Can you work these out from the model? Positions are in its coordinate system, mm. A direction names the side the tool comes from. Give positions to 0.01 mm unless a question says otherwise; leave off trailing zeros. Loops run counter-clockwise (first coordinate to the right, second up) from the corner with the lowest first, then second, coordinate; pieces in that order, holes last. Notation, with made-up numbers: M 49,33 L 91,33 A24 cw 91,52 Z; hole C 25.5,86 d8. An arc over 180 degrees is marked long. Answer as a JSON object with one key per item and string values.
```python
from build123d import *

# Parameters (mm, degrees)
SKETCH1_W           = 16.65
SKETCH1_H           = 12
BOSS_EXTRUDE1_DEPTH = 13
SKETCH2_W           = 7
SKETCH2_H           = 10.524951481
CUT_EXTRUDE1_DEPTH  = 13
SKETCH3_W           = 6.35563947
SKETCH3_H           = 6.957033312
SKETCH3_W_2         = 6.600584973
SKETCH3_H_2         = 6.806684851
BOSS_EXTRUDE2_DEPTH = 1
SKETCH4_R           = 2.546367572
SKETCH4_R_2         = 2.582102571
BOSS_EXTRUDE3_DEPTH = 1.5
FILLET1_R           = 1


with BuildPart() as part:
    # Sketch1 → Boss-Extrude1 (new body)
    with BuildSketch(Plane(origin=(0, 0, 0), x_dir=(1, 0, 0), z_dir=(0, 1, 0))):
        with Locations((-0.458958652, 0.629402757)):
            Rectangle(SKETCH1_W, SKETCH1_H)
    extrude(amount=BOSS_EXTRUDE1_DEPTH)

    # Sketch2 → Cut-Extrude1 (cut)
    with BuildSketch(Plane.XY.offset(5.370597243)):
        with Locations((-4.283958652, 12.062475741)):
            Rectangle(SKETCH2_W, SKETCH2_H)
        with Locations((3.366041348, 12.062475741)):
            Rectangle(SKETCH2_W, SKETCH2_H)
    extrude(amount=-CUT_EXTRUDE1_DEPTH, mode=Mode.SUBTRACT)

    # Sketch3 → Boss-Extrude2 (add)
    with BuildSketch(Plane(origin=(0, 6.8, 0), x_dir=(1, 0, 0), z_dir=(0, 1, 0))):
        with Locations((-4.190334083, 0.759249154)):
            Rectangle(SKETCH3_W, SKETCH3_H)
        with Locations((3.300292487, 0.834423384)):
            Rectangle(SKETCH3_W_2, SKETCH3_H_2)
    extrude(amount=BOSS_EXTRUDE2_DEPTH)

    # Sketch4 → Boss-Extrude3 (add)
    with BuildSketch(Plane(origin=(0, 7.8, 0), x_dir=(1, 0, 0), z_dir=(0, 1, 0))):
        with Locations((-4.183500062, 0.684074924)):
            Circle(SKETCH4_R)
        with Locations((3.456935343, 0.793419259)):
            Circle(SKETCH4_R_2)
    extrude(amount=BOSS_EXTRUDE3_DEPTH)

    # Fillet1
    fillet1_edges = [part.edges().sort_by_distance(p)[0] for p in [
        (-6.729867634, 9.3, -0.684074924),
        (0.874832772, 9.3, -0.793419259),
    ]]
    fillet(fillet1_edges, radius=FILLET1_R)


solid = part.part
```
1) Suppose I cut it at A-A, the plane y = 10.5. Write out the boundary of the cut face in (x, z), and give its area (3 significant figures).
Answer list:
{"outline": "M -8.78,-6.63 L -7.78,-6.63 L -7.78,5.37 L -8.78,5.37 Z; M -0.78,-6.63 L -0.13,-6.63 L -0.13,5.37 L -0.78,5.37 Z; M 6.87,-6.63 L 7.87,-6.63 L 7.87,5.37 L 6.87,5.37 Z", "area": "31.8 mm^2"}
2) For faces 1 (the flat face through (-4, 7, -4.238)), 2 (the flat face through (-0.134, 10, -1)), 3 (the cylindrical face through (-6.727, 8.046, -0.796)), 4 (the flat face through (-8, 13, -1)), 5 (the flat face through (3, 7, 2.569)), which set-ups out of +Z, -Z, +X, -X, +Y, -Y let a thin tool reach every point of the face, with its end or its side?
Answer list:
{"face 1": "-Z, +Y", "face 2": "+Z, -Z, +Y", "face 3": "+Y", "face 4": "+Z, -Z, +X, -X, +Y", "face 5": "+Z, +Y"}
3) Will these pins go through, and if not, where does the flat tip stop? pin 1 Ø0.9 at (x, z) = (3.5, -0.5) entering from +Y; pin 2 Ø1.1 at (x, y) = (-4.5, 7.5) entering from +Z.
Answer list:
{"pin 1": "y = 9.3", "pin 2": "z = 2.72"}
4) Suppose I cut it at C-C, the plane y = 9. Write out the boundary of the cut face in (x, z).
Answer list:
{"outline": "M -8.78,-6.63 L -7.78,-6.63 L -7.78,5.37 L -8.78,5.37 Z; C -4.18,-0.68 d4.52; M -0.78,-6.63 L -0.13,-6.63 L -0.13,5.37 L -0.78,5.37 Z; C 3.46,-0.79 d4.59; M 6.87,-6.63 L 7.87,-6.63 L 7.87,5.37 L 6.87,5.37 Z"}
5) If we mould it in two halves opening along X, with no side actions, what happens to faces 6 (the flat face through (-8.784, 6, -1)), 7 (the flat face through (7.4, 13, -0.7)), 8 (the flat face through (-0.784, 10, -1)), 9 (the flat face through (7.866, 6, -1))? For each: +X half, -X half, draft (parallel to the pull), parting line (faces both ways), or undercut.
Answer list:
{"face 6": "-X half", "face 7": "draft", "face 8": "undercut", "face 9": "+X half"}
6) Suppose I cut it at B-B, the plane z = -5.75. Write out the boundary of the cut face in (x, y), and give its area (3 significant figures).
Answer list:
{"outline": "M -8.78,0 L 7.87,0 L 7.87,13 L 6.87,13 L 6.87,6.8 L -0.13,6.8 L -0.13,13 L -0.78,13 L -0.78,6.8 L -7.78,6.8 L -7.78,13 L -8.78,13 Z", "area": "130 mm^2"}
7) Please list where these lines run through material, in increasing order: line 1 along X through (y, z) = (11, 3); line 2 along Y through (x, z) = (0.25, 3.75); line 3 along Y through (x, z) = (-6.25, -2.25). Write a range as from..to.
Answer list:
{"line 1": "-8.78..-7.78, -0.78..-0.13, 6.87..7.87", "line 2": "0..6.8", "line 3": "0..7.8"}
